Design review of the part built by this model. Coordinates are the model's own, in mm. Face numbers are marked on the shaded views. A direction names the side the tool comes from. Coordinates: 2 decimals unless noted, no trailing zeros. Loops run counter-clockwise (first coordinate to the right, second up) from the corner with the lowest first, then second, coordinate; pieces in that order, holes last.
Q1. Machinability: for the marked faces 1 and 2, which of the approach directions +Z, -Z, +X, -X, +Y, -Y give a long, thin tool a straight path to every point of the face, cutting with its end or side? Answer none if there is none.
Q2. Wall thickness on probe 1 along X at (y, z) = (0.75, 4.75); probe 2 along X at (y, z) = (1.55, -7.75); probe 3 along X at (y, z) = (1.2, 8): over which ranges is each line inside the solid? List them lowest first.
Q3. Add section B-B on x = 0. Give the boundary of the cut face in (y, z) (3 decimals), and give its area (3 significant figures).
Q4. Add section A-A on z = 0. Give the boundary of the cut face in (x, y) (3 decimals).
Q5. Draft analysis for pull direction Z (two halves, no side actions). For the marked faces 3, 4 and 5, state which applies: released by +Z, released by -Z, zero draft, split by the parting line, or undercut.
Q6. For P1, Ø0.8, axis at x = -0.5, y = 1, coming from the -Z side; P2, Ø0.6, axis at x = -8.5, y = 1.5, coming from the +Z side; P3, Ø1.5, axis at x = -10, y = 0.5, coming from the +Z side; P4, Ø1.7, axis at y = 1.5, z = -8.5, coming from the -X side, all flat-tipped, find the tip position at first contact; note any pin that passes through.
Q7. Add section D-D on x = 8. Give the boundary of the cut face in (y, z).
Q8. Add section C-C on y = 2.55. Give the boundary of the cut face in (x, z), and give its area (3 significant figures).
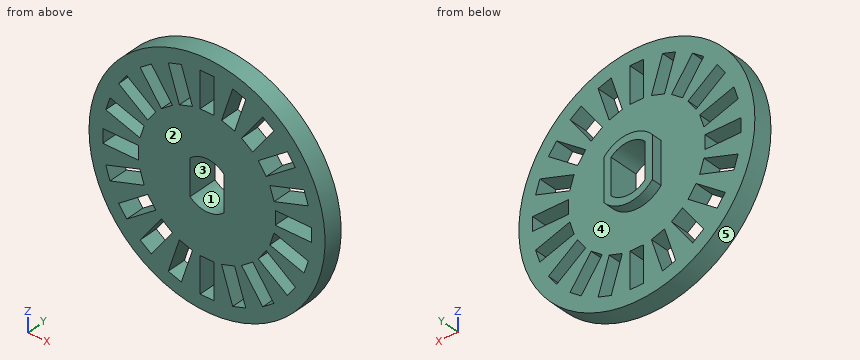
Autodesk Inventor part; units mm, degrees
ref_plane "YZ Plane" through (0, 0, 0) normal (1, 0, 0) x (0, 1, 0)
ref_plane "XZ Plane" through (0, 0, 0) normal (0, 1, 0) x (-1, 0, 0)
ref_plane "XY Plane" through (0, 0, 0) normal (0, 0, 1) x (1, 0, 0)
sketch "Sketch1" plane through (0, 0, 0) normal (0, 1, 0) x (-1, 0, 0)
  circle A0 centre (0, 0) radius 12.875
  arc A1 (-1.85, -1.9666) -> (1.85, -1.9666) centre (0, 0) ccw
  line L0 (1.85, 1.9666) -> (1.85, -1.9666)
  line L1 (-1.85, 1.9666) -> (-1.85, -1.9666)
  line L2 (7.45, 0.75) -> (11.375, 0.75)
  line L3 (11.375, 0.75) -> (11.375, -0.75)
  line L4 (11.375, -0.75) -> (7.45, -0.75)
  line L5 (7.45, -0.75) -> (7.45, 0.75)
  line L6 (0, 0) -> (11.375, 0) construction
  line L7 (11.05, 2.8018) -> (7.3171, 1.5889)
  line L8 (10.5865, 4.2284) -> (11.05, 2.8018)
  line L9 (6.8536, 3.0155) -> (10.5865, 4.2284)
  line L10 (7.3171, 1.5889) -> (6.8536, 3.0155)
  line L11 (9.6434, 6.0793) -> (6.468, 3.7722)
  line L12 (8.7617, 7.2928) -> (9.6434, 6.0793)
  line L13 (5.5863, 4.9858) -> (8.7617, 7.2928)
  line L14 (6.468, 3.7722) -> (5.5863, 4.9858)
  line L15 (7.2928, 8.7617) -> (4.9858, 5.5863)
  line L16 (6.0793, 9.6434) -> (7.2928, 8.7617)
  line L17 (3.7722, 6.468) -> (6.0793, 9.6434)
  line L18 (4.9858, 5.5863) -> (3.7722, 6.468)
  line L19 (4.2284, 10.5865) -> (3.0155, 6.8536)
  line L20 (2.8018, 11.05) -> (4.2284, 10.5865)
  line L21 (1.5889, 7.3171) -> (2.8018, 11.05)
  line L22 (3.0155, 6.8536) -> (1.5889, 7.3171)
  line L23 (0.75, 11.375) -> (0.75, 7.45)
  line L24 (-0.75, 11.375) -> (0.75, 11.375)
  line L25 (-0.75, 7.45) -> (-0.75, 11.375)
  line L26 (0.75, 7.45) -> (-0.75, 7.45)
  line L27 (-2.8018, 11.05) -> (-1.5889, 7.3171)
  line L28 (-4.2284, 10.5865) -> (-2.8018, 11.05)
  line L29 (-3.0155, 6.8536) -> (-4.2284, 10.5865)
  line L30 (-1.5889, 7.3171) -> (-3.0155, 6.8536)
  line L31 (-6.0793, 9.6434) -> (-3.7722, 6.468)
  line L32 (-7.2928, 8.7617) -> (-6.0793, 9.6434)
  line L33 (-4.9858, 5.5863) -> (-7.2928, 8.7617)
  line L34 (-3.7722, 6.468) -> (-4.9858, 5.5863)
  line L35 (-8.7617, 7.2928) -> (-5.5863, 4.9858)
  line L36 (-9.6434, 6.0793) -> (-8.7617, 7.2928)
  line L37 (-6.468, 3.7722) -> (-9.6434, 6.0793)
  line L38 (-5.5863, 4.9858) -> (-6.468, 3.7722)
  line L39 (-10.5865, 4.2284) -> (-6.8536, 3.0155)
  line L40 (-11.05, 2.8018) -> (-10.5865, 4.2284)
  line L41 (-7.3171, 1.5889) -> (-11.05, 2.8018)
  line L42 (-6.8536, 3.0155) -> (-7.3171, 1.5889)
  line L43 (-11.375, 0.75) -> (-7.45, 0.75)
  line L44 (-11.375, -0.75) -> (-11.375, 0.75)
  line L45 (-7.45, -0.75) -> (-11.375, -0.75)
  line L46 (-7.45, 0.75) -> (-7.45, -0.75)
  line L47 (-11.05, -2.8018) -> (-7.3171, -1.5889)
  line L48 (-10.5865, -4.2284) -> (-11.05, -2.8018)
  line L49 (-6.8536, -3.0155) -> (-10.5865, -4.2284)
  line L50 (-7.3171, -1.5889) -> (-6.8536, -3.0155)
  line L51 (-9.6434, -6.0793) -> (-6.468, -3.7722)
  line L52 (-8.7617, -7.2928) -> (-9.6434, -6.0793)
  line L53 (-5.5863, -4.9858) -> (-8.7617, -7.2928)
  line L54 (-6.468, -3.7722) -> (-5.5863, -4.9858)
  line L55 (-7.2928, -8.7617) -> (-4.9858, -5.5863)
  line L56 (-6.0793, -9.6434) -> (-7.2928, -8.7617)
  line L57 (-3.7722, -6.468) -> (-6.0793, -9.6434)
  line L58 (-4.9858, -5.5863) -> (-3.7722, -6.468)
  line L59 (-4.2284, -10.5865) -> (-3.0155, -6.8536)
  line L60 (-2.8018, -11.05) -> (-4.2284, -10.5865)
  line L61 (-1.5889, -7.3171) -> (-2.8018, -11.05)
  line L62 (-3.0155, -6.8536) -> (-1.5889, -7.3171)
  line L63 (-0.75, -11.375) -> (-0.75, -7.45)
  line L64 (0.75, -11.375) -> (-0.75, -11.375)
  line L65 (0.75, -7.45) -> (0.75, -11.375)
  line L66 (-0.75, -7.45) -> (0.75, -7.45)
  line L67 (2.8018, -11.05) -> (1.5889, -7.3171)
  line L68 (4.2284, -10.5865) -> (2.8018, -11.05)
  line L69 (3.0155, -6.8536) -> (4.2284, -10.5865)
  line L70 (1.5889, -7.3171) -> (3.0155, -6.8536)
  line L71 (6.0793, -9.6434) -> (3.7722, -6.468)
  line L72 (7.2928, -8.7617) -> (6.0793, -9.6434)
  line L73 (4.9858, -5.5863) -> (7.2928, -8.7617)
  line L74 (3.7722, -6.468) -> (4.9858, -5.5863)
  line L75 (8.7617, -7.2928) -> (5.5863, -4.9858)
  line L76 (9.6434, -6.0793) -> (8.7617, -7.2928)
  line L77 (6.468, -3.7722) -> (9.6434, -6.0793)
  line L78 (5.5863, -4.9858) -> (6.468, -3.7722)
  line L79 (10.5865, -4.2284) -> (6.8536, -3.0155)
  line L80 (11.05, -2.8018) -> (10.5865, -4.2284)
  line L81 (7.3171, -1.5889) -> (11.05, -2.8018)
  line L82 (6.8536, -3.0155) -> (7.3171, -1.5889)
  arc A2 (-1.85, 1.9666) -> (-1.85, -1.9666) centre (0, 0) ccw construction
  arc A3 (1.85, 1.9666) -> (-1.85, 1.9666) centre (0, 0) ccw
  arc A4 (1.85, -1.9666) -> (1.85, 1.9666) centre (0, 0) ccw construction
  point P0 (10.8183, 3.5151)
  point P1 (9.2026, 6.6861)
  point P2 (6.6861, 9.2026)
  point P3 (3.5151, 10.8183)
  point P4 (0, 11.375)
  point P5 (-3.5151, 10.8183)
  point P6 (-6.6861, 9.2026)
  point P7 (-9.2026, 6.6861)
  point P8 (-10.8183, 3.5151)
  point P9 (-11.375, 0)
  point P10 (-10.8183, -3.5151)
  point P11 (-9.2026, -6.6861)
  point P12 (-6.6861, -9.2026)
  point P13 (-3.5151, -10.8183)
  point P14 (0, -11.375)
  point P15 (3.5151, -10.8183)
  point P16 (6.6861, -9.2026)
  point P17 (9.2026, -6.6861)
  point P18 (10.8183, -3.5151)
  dimension "d0" = 25.75
  dimension "d1" = 5.4
  dimension "d3" = 3.7
  dimension "d4" = 4.75
  dimension "d5" = 1.5
  dimension "d6" = 1.5
  dimension "d9" = 360
extrude "Extrusion1" add sketch "Sketch1" along normal blind 2.1
sketch "Sketch2" plane through (0, 2.1, 0) normal (0, 1, 0) x (1, 0, 0)
  arc A0 (1.85, 1.9666) -> (-1.85, 1.9666) centre (0, 0) ccw
  line L0 (1.85, 1.9666) -> (1.85, -1.9666)
  arc A1 (-1.85, -1.9666) -> (1.85, -1.9666) centre (0, 0) ccw
  line L1 (-1.85, -1.9666) -> (-1.85, 1.9666)
  arc A2 (-2.65, -2.2864) -> (2.65, -2.2864) centre (0, 0) ccw
  arc A3 (2.65, 2.2864) -> (-2.65, 2.2864) centre (0, 0) ccw
  line L2 (-2.65, -2.2864) -> (-2.65, 2.2864)
  line L3 (2.65, 2.2864) -> (2.65, -2.2864)
  dimension "d13" = 0.8
  dimension "d14" = 0.8
  dimension "d15" = 0.8
extrude "Extrusion2" add sketch "Sketch2" along normal blind 1.15
properties part number "TT encoder disk"
Entries:
1. face 1: +Y, -Y
1. face 2: +Z, -Z, +X, -X, -Y
2. probe 1: x = -11.97 to -7.81, -5.76 to 5.76, 7.81 to 11.97
2. probe 2: x = -10.28 to -6.56, -4.7 to -3.31, -1.73 to -0.75, 0.75 to 1.73, 3.31 to 4.7, 6.56 to 10.28
2. probe 3: x = -10.09 to -6.74, -4.89 to -3.39, -1.81 to -0.75, 0.75 to 1.81, 3.39 to 4.89, 6.74 to 10.09
3. outline: (0, -12.875) - (2.1, -12.875) - (2.1, -11.375) - (0, -11.375) - close; (0, -7.45) - (2.1, -7.45) - (2.1, -3.5) - (3.25, -3.5) - (3.25, -2.7) - (0, -2.7) - close; (0, 2.7) - (3.25, 2.7) - (3.25, 3.5) - (2.1, 3.5) - (2.1, 7.45) - (0, 7.45) - close; (0, 11.375) - (2.1, 11.375) - (2.1, 12.875) - (0, 12.875) - close
3. area: 28.1 mm2
4. outline: (-12.875, 0) - (-11.375, 0) - (-11.375, 2.1) - (-12.875, 2.1) - close; (-7.45, 0) - (-1.85, 0) - (-1.85, 3.25) - (-2.65, 3.25) - (-2.65, 2.1) - (-7.45, 2.1) - close; (1.85, 0) - (7.45, 0) - (7.45, 2.1) - (2.65, 2.1) - (2.65, 3.25) - (1.85, 3.25) - close; (11.375, 0) - (12.875, 0) - (12.875, 2.1) - (11.375, 2.1) - close
5. face 3: undercut
5. face 4: zero draft
5. face 5: split by the parting line
6. P1: stops at z = -12.87
6. P2: stops at z = 9.93
6. P3: stops at z = 8.96
6. P4: stops at x = -10.36
7. outline: (0, -10.09) - (2.1, -10.09) - (2.1, -6.74) - (0, -6.74) - close; (0, -4.89) - (2.1, -4.89) - (2.1, -3.39) - (0, -3.39) - close; (0, -1.81) - (2.1, -1.81) - (2.1, -0.75) - (0, -0.75) - close; (0, 0.75) - (2.1, 0.75) - (2.1, 1.81) - (0, 1.81) - close; (0, 3.39) - (2.1, 3.39) - (2.1, 4.89) - (0, 4.89) - close; (0, 6.74) - (2.1, 6.74) - (2.1, 10.09) - (0, 10.09) - close
8. outline: (-2.65, -2.29) arc R3.5 ccw to (2.65, -2.29) - (2.65, 2.29) arc R3.5 ccw to (-2.65, 2.29) - close; hole (-1.85, -1.97) arc R2.7 ccw to (1.85, -1.97) - (1.85, 1.97) arc R2.7 ccw to (-1.85, 1.97) - close
8. area: 14.9 mm2
